Verification items for the finished model (mm, model axes). Round coordinates to 2 decimals unless told otherwise and drop trailing zeros. Loops run counter-clockwise (first coordinate to the right, second up) from the corner with the lowest first, then second, coordinate; pieces in that order, holes last. Notation, with made-up numbers: (85, 25) - (116, 25) arc R22 cw to (116, 39) - close; hole circle Ø11 at (38, 5.25). An arc over 180 degrees is marked (long way). Use a Markdown table: item, result. Add a question column.
```python
from build123d import *

# Parameters (mm, degrees)
ESQUISSE2_R        = 1.08
BOSS_EXTRU_1_DEPTH = 0.15


with BuildPart() as part:
    # Esquisse1 → Révolution1 (revolve)
    with BuildSketch(Plane.XY):
        Polygon((-1.23, 0), (-1.23, 0.3), (-1.08, 0.3), (-1.08, 0.45), (-1.13245676, 0.567603094), (-1.030107007, 0.6), (-0.93, 0.6), (-0.93, 0), align=None)
    revolve(axis=Axis((0, 0, 0), (0, 1, 0)))

    # Esquisse2 → Boss.-Extru.1 (add)
    with BuildSketch(Plane(origin=(0, 0.3, 0), x_dir=(1, 0, 0), z_dir=(0, 1, 0))):
        with BuildLine():
            Line((0.099960806, 12.002799494), (0.4, 1.289379696))
            ThreePointArc((0.4, 1.289379696), (1.338815312, 0.173417305), (0.715314881, -1.144912495))
            ThreePointArc((0.715314881, -1.144912495), (0.539593784, -1.332680285), (0.480442286, -1.582951632))
            Line((0.480442286, -1.582951632), (0.48324178, -1.682912439))
            ThreePointArc((0.48324178, -1.682912439), (0.531110798, -1.882818549), (0.655363875, -2.04657162))
            ThreePointArc((0.655363875, -2.04657162), (0, -3.801884927), (-0.655363875, -2.04657162))
            ThreePointArc((-0.655363875, -2.04657162), (-0.531110798, -1.882818549), (-0.48324178, -1.682912439))
            Line((-0.48324178, -1.682912439), (-0.480442286, -1.582951632))
            ThreePointArc((-0.480442286, -1.582951632), (-0.539593784, -1.332680285), (-0.715314881, -1.144912495))
            ThreePointArc((-0.715314881, -1.144912495), (-1.338815312, 0.173417305), (-0.4, 1.289379696))
            Line((-0.4, 1.289379696), (-0.099960806, 12.002799494))
            ThreePointArc((-0.099960806, 12.002799494), (0, 12.1), (0.099960806, 12.002799494))
        make_face()
        Circle(ESQUISSE2_R, mode=Mode.SUBTRACT)
    extrude(amount=BOSS_EXTRU_1_DEPTH)


solid = part.part
```
Q1. Section check D-D on z = -5.5. Record the cut outline in (x, y).
Q2. Section check A-A on z = 0. Record the cut outline in (x, y), plus the area to 3 significant figures.
Q3. Go/stop test with a flat-tipped pin: pin 1 Ø0.8 at (x, z) = (0.5, -3.5) entering from +Y. Record where the tip stops, or that it passes through.
Q4. Section check C-C on z = -10.75. Record the cut outline in (x, y).
Q5. Thickness scan on line 1 along Z through (x, y) = (-0.05, 0.15); line 2 along Z through (x, y) = (-0.45, 0.1); line 3 along X through (y, z) = (0.2, -0.5). Record the ranges inside material, lowest first.
Q6. Section check B-B on y = 0.1. Record the cut outline in (x, z), plus the area to 3 significant figures.
Determined:
| question | item | result |
|---|---|---|
| 1 | outline | (-0.28, 0.3) - (0.28, 0.3) - (0.28, 0.45) - (-0.28, 0.45) - close |
| 2 | outline | (-1.35, 0.3) - (-1.23, 0.3) - (-1.23, 0) - (-0.93, 0) - (-0.93, 0.6) - (-1.03, 0.6) - (-1.13, 0.57) - (-1.08, 0.45) - (-1.35, 0.45) - close; (0.93, 0) - (1.23, 0) - (1.23, 0.3) - (1.35, 0.3) - (1.35, 0.45) - (1.08, 0.45) - (1.13, 0.57) - (1.03, 0.6) - (0.93, 0.6) - close |
| 2 | area | 0.357 mm² |
| 3 | pin 1 | stops at y = 0.45 |
| 4 | outline | (-0.14, 0.3) - (0.14, 0.3) - (0.14, 0.45) - (-0.14, 0.45) - close |
| 5 | line 1 | z = -1.23 to -0.93, 0.93 to 1.23 |
| 5 | line 2 | z = -1.14 to -0.81, 0.81 to 1.14 |
| 5 | line 3 | x = -1.12 to -0.78, 0.78 to 1.12 |
| 6 | outline | circle Ø2.46 at (0, 0); hole circle Ø1.86 at (0, 0) |
| 6 | area | 2.04 mm² |
